```python
from build123d import *

# Parameters (mm, degrees)
BASE_EXTRUDE_DEPTH      = 62.2325
BASE_EXTRUDE_DEPTH_BACK = 62.2325
SKETCH1_R               = 10.25
STROKECHAMBER_START     = -46.95
SKETCH2_R               = 9.525
STROKECHAMBER_DEPTH     = 93.9
RODBORE_DEPTH           = 64.898427651
RODBORE_DEPTH_BACK      = 64.898427651
SKETCH3_R               = 4
FILLET1_R               = 0.25
SKETCH4_R               = 9.55
CUT_EXTRUDE1_DEPTH      = 5


with BuildPart() as part:
    # Sketch1 → Base-Extrude (new, two sides: drawn at the far end of the back side and taken through both)
    with BuildSketch(Plane.XY.offset(-BASE_EXTRUDE_DEPTH_BACK)):
        Circle(SKETCH1_R)
    extrude(amount=BASE_EXTRUDE_DEPTH + BASE_EXTRUDE_DEPTH_BACK)

    # Sketch2 → StrokeChamber (cut)
    with BuildSketch(Plane.XY.offset(STROKECHAMBER_START)):
        Circle(SKETCH2_R)
    extrude(amount=STROKECHAMBER_DEPTH, mode=Mode.SUBTRACT)

    # Sketch3 → RodBore (cut, two sides: drawn at the far end of the back side and taken through both)
    with BuildSketch(Plane.XY.offset(-RODBORE_DEPTH_BACK)):
        Circle(SKETCH3_R)
    extrude(amount=RODBORE_DEPTH + RODBORE_DEPTH_BACK, mode=Mode.SUBTRACT)

    # Fillet1
    fillet1_edges = [part.edges().sort_by_distance(p)[0] for p in [
        (-10.25, 0, -62.2325),
        (-10.25, 0, 62.2325),
    ]]
    fillet(fillet1_edges, radius=FILLET1_R)

    # Sketch4 → Cut-Extrude1 (cut)
    with BuildSketch(Plane.XY.offset(62.2325)):
        Circle(SKETCH4_R)
    cut_extrude1 = extrude(amount=-CUT_EXTRUDE1_DEPTH, mode=Mode.SUBTRACT)

    # Mirror1: Cut-Extrude1 across plane
    add(cut_extrude1.mirror(Plane.XY), mode=Mode.SUBTRACT)


solid = part.part
```
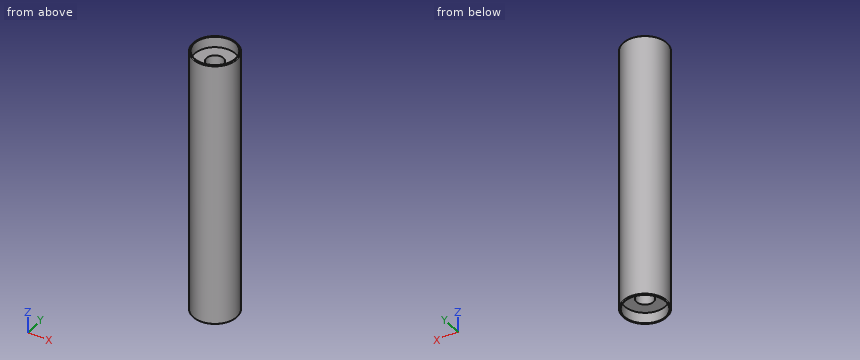
Geometry: final body of the model. Coordinates: model frame, mm. Round coordinates to 2 decimals unless told otherwise and drop trailing zeros. Order: outer loops, then holes, each group sorted by start corner. A loop starts at its lowest first (then second) coordinate and runs counter-clockwise, first axis right, second up. Notation, with made-up numbers: (27, -36.5) -> (47, -36.5) arc R22 cw to (47, -25.5) -> close; hole circle Ø10 at (87.25, 86.25). An arc over 180 degrees is marked (long way). Use CSV: the item, a comma, the result in double quotes. Start each with the question number.
1) Section C-C (z = -0.5). Return the cut outline in (x, y) (3 decimals).
2) Material intervals for line 1 along Z through (x, y) = (0.75, 5); line 2 along Y through (x, z) = (0, -59.05); line 3 along Y through (x, z) = (0, -53.25), sorted ascending. Write a range as from..to.
3) First-contact query: pin 1 Ø1.5 at (x, y) = (-2, -7.5) entering from -Z; pin 2 Ø3 at (x, z) = (8, -8.5) entering from +Y; pin 3 Ø8 at (x, z) = (-7, 38) entering from -Y; pin 4 Ø3 at (y, z) = (1.5, 32) entering from +X. Flat tips, straight axial feed; report the tip coordinate or a pass-through.
Returned:
1,outline,"circle Ø20.5 at (0, 0); hole circle Ø19.05 at (0, 0)"
2,line 1,"z = -57.23..-46.95, 46.95..57.23"
2,line 2,"y = -10.25..-9.55, 9.55..10.25"
2,line 3,"y = -10.25..-4, 4..10.25"
3,pin 1,"stops at z = -57.23"
3,pin 2,"stops at y = 7.93"
3,pin 3,"stops at y = -9.8"
3,pin 4,"stops at x = 10.25"
